```python
from build123d import *

# Parameters (mm, degrees)
SKETCH1_R           = 1.2499975
BOSS_EXTRUDE1_DEPTH = 1.5
SKETCH2_R           = 0.5
CUT_EXTRUDE1_DEPTH  = 1.5
SKETCH4_R           = 3.5
SKETCH4_R_2         = 2.5
BOSS_EXTRUDE2_DEPTH = 2.25
SKETCH5_R           = 2.5
SKETCH5_R_2         = 1.2499975
CUT_EXTRUDE2_DEPTH  = 0.75


with BuildPart() as part:
    # Sketch1 → Boss-Extrude1 (new body)
    with BuildSketch(Plane.XY):
        with BuildLine():
            Line((-1.994891435, 14.142857143), (-2.863567464, 2.012456554))
            ThreePointArc((-2.863567464, 2.012456554), (-3.5, 0), (-2.863567464, -2.012456554))
            Line((-2.863567464, -2.012456554), (-1.994891435, -14.142857143))
            ThreePointArc((-1.994891435, -14.142857143), (0, -16), (1.994891435, -14.142857143))
            Line((1.994891435, -14.142857143), (2.863567464, -2.012456554))
            ThreePointArc((2.863567464, -2.012456554), (3.5, 0), (2.863567464, 2.012456554))
            Line((2.863567464, 2.012456554), (1.994891435, 14.142857143))
            ThreePointArc((1.994891435, 14.142857143), (0, 16), (-1.994891435, 14.142857143))
        make_face()
        Circle(SKETCH1_R, mode=Mode.SUBTRACT)
    extrude(amount=BOSS_EXTRUDE1_DEPTH)

    # Sketch2 → Cut-Extrude1 (cut)
    with BuildSketch(Plane.XY.offset(1.5)):
        with Locations((0, 10.5)):
            Circle(SKETCH2_R)
        with Locations((0, -10.5)):
            Circle(SKETCH2_R)
    extrude(amount=-CUT_EXTRUDE1_DEPTH, mode=Mode.SUBTRACT)

    # Sketch4 → Boss-Extrude2 (add)
    with BuildSketch(Plane(origin=(0, 0, 0), x_dir=(-1, 0, 0), z_dir=(0, 0, -1))):
        Circle(SKETCH4_R)
        Circle(SKETCH4_R_2, mode=Mode.SUBTRACT)
    extrude(amount=BOSS_EXTRUDE2_DEPTH)

    # Sketch5 → Cut-Extrude2 (cut)
    with BuildSketch(Plane.XY.offset(1.5)):
        Circle(SKETCH5_R)
        Circle(SKETCH5_R_2, mode=Mode.SUBTRACT)
    extrude(amount=-CUT_EXTRUDE2_DEPTH, mode=Mode.SUBTRACT)


solid = part.part
```
Can you work these out from the model? Positions are in its coordinate system, mm. A direction names the side the tool comes from. Coordinates: 2 decimals unless noted, no trailing zeros. Write each loop counter-clockwise with the first axis right and the second up, starting at its lowest first coordinate (ties: lowest second). Pieces come first, ordered by that corner, then holes. Notation, with made-up numbers: (51, 56.5) - (94, 56.5) arc R13 ccw to (94, 66.5) - close; hole circle Ø7 at (1, -32.5). An arc over 180 degrees is marked (long way). Return JSON: item names as keys, results as strings.
Q1. If we section it at B-B (z = -1.4): Please give me the cut outline in (x, y).
Computed values:
{"outline": "circle Ø7 at (0, 0); hole circle Ø5 at (0, 0)"}
Q2. If we section it at C-C (y = 10.5): Please give me the cut outline in (x, z).
Computed values:
{"outline": "(-2.26, 0) - (-0.5, 0) - (-0.5, 1.5) - (-2.26, 1.5) - close; (0.5, 0) - (2.26, 0) - (2.26, 1.5) - (0.5, 1.5) - close"}
Q3. On a 3-axis mill with a long thin cutter (end or side, diameter ignored), from which of +Z, -Z, +X, -X, +Y, -Y can I reach the whole of each face in a straight line? I mean faces 5 (the flat face through (-2.423, 8.163, 0.74)), 6 (the cylindrical face through (0.54, -2.44, -1.11)), 7 (the flat face through (-1, -1, 0.75)). Say none if no direction works.
Computed values:
{"face 5": "+Z, -Z, -X, +Y", "face 6": "-Z", "face 7": "+Z"}
Q4. Thinking about a two-plate mould opening in X: for faces 1 (the flat face through (-2.435, -7.993, 0.74)), 2 (the flat face through (3, 0, 1.5)), 3 (the cylindrical face through (0, 16, 1)), 4 (the flat face through (1, 1, 0)), which applies, +X half, -X half, draft (parallel to the pull), parting line (faces both ways), or undercut?
Computed values:
{"face 1": "-X half", "face 2": "draft", "face 3": "parting line", "face 4": "undercut"}
Q5. I'm going to push flat-ended pins straight in: pin 1 Ø2.5 at (x, y) = (-1, 0.5) entering from +Z; pin 2 Ø3 at (x, y) = (-2, 10) entering from -Z; pin 3 Ø1.5 at (x, y) = (0, 0) entering from -Z (3 decimals). Where does each tip first touch, or does it pass through?
Computed values:
{"pin 1": "stops at z = 0.75", "pin 2": "stops at z = 0", "pin 3": "passes through"}
Q6. If we section it at D-D (y = 4.5): Please give me the cut outline in (x, z), then the cut area to 3 significant figures.
Computed values:
{"outline": "(-2.69, 0) - (2.69, 0) - (2.69, 1.5) - (-2.69, 1.5) - close", "area": "8.06 mm2"}
Q7. If we section it at A-A (y = 0): Please give me the cut outline in (x, z).
Computed values:
{"outline": "(-3.5, -2.25) - (-2.5, -2.25) - (-2.5, 0) - (-1.25, 0) - (-1.25, 0.75) - (-2.5, 0.75) - (-2.5, 1.5) - (-3.5, 1.5) - close; (1.25, 0) - (2.5, 0) - (2.5, -2.25) - (3.5, -2.25) - (3.5, 1.5) - (2.5, 1.5) - (2.5, 0.75) - (1.25, 0.75) - close"}
Q8. Please list where these lines run through material, in increasing order: L1, parallel to X at y = 7, z = 1.05; L2, parallel to Z at x = 1, y = 7.5; L3, parallel to Y at x = -0.75, z = -1.3. Write a range as from..to.
Computed values:
{"L1": "x = -2.51..2.51", "L2": "z = 0..1.5", "L3": "y = -3.42..-2.38, 2.38..3.42"}
